from build123d import *

# Parameters (mm, degrees)
SKETCH1_R           = 62.5
BOSS_EXTRUDE1_DEPTH = 450
SCALE1_SCALE        = 2


with BuildPart() as part:
    # Sketch1 → Boss-Extrude1 (new body)
    with BuildSketch(Plane.XY):
        with BuildLine():
            ThreePointArc((0, 82.5), (-125.896146437, 125.896146437), (-82.5, 0))
            ThreePointArc((-82.5, 0), (-125.896146437, -125.896146437), (0, -82.5))
            ThreePointArc((0, -82.5), (125.896146437, -125.896146437), (82.5, 0))
            ThreePointArc((82.5, 0), (125.896146437, 125.896146437), (0, 82.5))
        make_face()
        with BuildLine():
            ThreePointArc((-20.204468067, -82.5), (-112.61028354, -110.878115832), (-80.075757576, -19.85253255))
            Line((-80.075757576, -19.85253255), (-23.459201006, -79.094348016))
            ThreePointArc((-23.459201006, -79.094348016), (-21.661425556, -79.605481237), (-19.85253255, -80.075757576))
            ThreePointArc((-19.85253255, -80.075757576), (-20.014769218, -81.289872177), (-20.204468067, -82.5))
        make_face(mode=Mode.SUBTRACT)
        with BuildLine():
            ThreePointArc((80.075757576, -19.85253255), (111.754010814, -111.754010814), (19.85253255, -80.075757576))
            Line((19.85253255, -80.075757576), (80.075757576, -19.85253255))
        make_face(mode=Mode.SUBTRACT)
        Circle(SKETCH1_R, mode=Mode.SUBTRACT)
        with BuildLine():
            ThreePointArc((-80.075757576, 19.85253255), (-111.754010814, 111.754010814), (-19.85253255, 80.075757576))
            Line((-19.85253255, 80.075757576), (-80.075757576, 19.85253255))
        make_face(mode=Mode.SUBTRACT)
        with BuildLine():
            ThreePointArc((19.85253255, 80.075757576), (111.754010814, 111.754010814), (80.075757576, 19.85253255))
            Line((80.075757576, 19.85253255), (19.85253255, 80.075757576))
        make_face(mode=Mode.SUBTRACT)
    extrude(amount=BOSS_EXTRUDE1_DEPTH)


with BuildPart() as part_1:
    # Scale1: scaled about (-0.110996519, -0.161131332, 225)
    add(part.part.scale(SCALE1_SCALE).moved(Location((0.110996519, 0.161131332, -225))))


solid = part_1.part
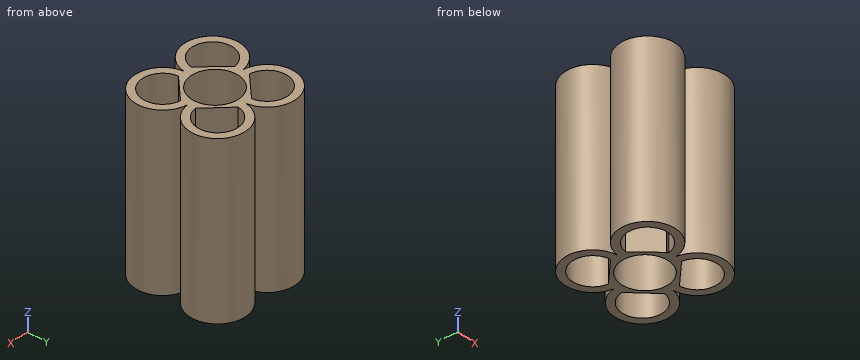
Source: CAD feature listing. Evaluate the final solid. Frame: model axes, mm. Round coordinates to 2 decimals unless told otherwise and drop trailing zeros. Loops run counter-clockwise (first coordinate to the right, second up) from the corner with the lowest first, then second, coordinate; pieces in that order, holes last. Notation, with made-up numbers: (7, -15.5) - (27, -15.5) arc R23 cw to (27, 11.5) - close; hole circle Ø9 at (29.25, 78). An arc over 180 degrees is marked (long way). Write item = value, one per line. Start each with the question number.
(1) Section query C-C, the plane x = 146.5. Output: boundary loops of the cut face in (y, z), plus the area to 3 significant figures.
(2) Section query B-B, the plane x = 77.5. Output: boundary loops of the cut face in (y, z), plus the area to 3 significant figures.
(3) Section query A-A, the plane y = 192. Output: boundary loops of the cut face in (x, z), plus the area to 3 significant figures.
(4) Ray query, line 1 along X through (y, z) = (-84, 361.5); line 2 along Y through (x, z) = (78.5, -84.5) (3 decimals); line 3 along Y through (x, z) = (-183.5, -3). Return the intervals inside material, ascending. Write a range as from..to.
(5) Section query D-D, the plane y = -27.5. Output: boundary loops of the cut face in (x, z), plus the area to 3 significant figures.
(6) Pin query (flat end, axial travel): pin 1 (8 mm diameter, centred on x = 188.5, z = -131.5, fed in from -Y); pin 2 (1.5 mm diameter, centred on x = 76, z = -131.5, fed in from +Y); pin 3 (12 mm diameter, centred on y = 111.5, z = 584, fed in from +X). Return the tip coordinate at first contact, or that it passes through.
Conclusion:
q1.outline = (-295.02, -225) - (-255.02, -225) - (-255.02, 675) - (-295.02, 675) - close; (-53.31, -225) - (53.63, -225) - (53.63, 675) - (-53.31, 675) - close; (255.34, -225) - (295.34, -225) - (295.34, 675) - (255.34, 675) - close
q1.area = 168,000 mm2
q2.outline = (-277.62, -225) - (-229.6, -225) - (-229.6, 675) - (-277.62, 675) - close; (-122.31, -225) - (-98, -225) - (-98, 675) - (-122.31, 675) - close; (98.32, -225) - (122.63, -225) - (122.63, 675) - (98.32, 675) - close; (229.92, -225) - (277.94, -225) - (277.94, 675) - (229.92, 675) - close
q2.area = 130,000 mm2
q3.outline = (-288.13, -225) - (-245.36, -225) - (-245.36, 675) - (-288.13, 675) - close; (-48.51, -225) - (-5.73, -225) - (-5.73, 675) - (-48.51, 675) - close; (5.95, -225) - (48.73, -225) - (48.73, 675) - (5.95, 675) - close; (245.58, -225) - (288.36, -225) - (288.36, 675) - (245.58, 675) - close
q3.area = 154,000 mm2
q4.line_1 = -281.06..-234.91, -117.55..-92.31, 92.53..115.81, 235.13..281.28
q4.line_2 = -278.149..-230.429, -121.306..-97.205, 97.527..121.629, 230.751..278.472
q4.line_3 = -290.44..-248.65, -45.12..-3.33, 3.65..45.44, 248.97..290.76
q5.outline = (-234.64, -225) - (-121.79, -225) - (-121.79, 675) - (-234.64, 675) - close; (122.01, -225) - (234.86, -225) - (234.86, 675) - (122.01, 675) - close
q5.area = 203,000 mm2
q6.pin_1 = -290.23
q6.pin_2 = 277.54
q6.pin_3 = 292.28
